Check sheet for the modelled part. Datum: model origin and axes. Units: mm. A direction names the side the tool comes from. Coordinates: 2 decimals unless noted, no trailing zeros. Write each loop counter-clockwise with the first axis right and the second up, starting at its lowest first coordinate (ties: lowest second). Pieces come first, ordered by that corner, then holes. Notation, with made-up numbers: (67.25, -38.75) -> (123.25, -38.75) arc R23 ccw to (123.25, -4.75) -> close; hole circle Ø11 at (-9, -38). An arc over 180 degrees is marked (long way). Put each result on its own line as item: value.
```python
from build123d import *

# Parameters (mm, degrees)
ESQUISSE1_W                  = 20
ESQUISSE1_H                  = 12
BOSS_EXTRU_1_DEPTH           = 15
ESQUISSE1_4_R                = 4.2
ENL_V_MAT_EXTRU_1_DEPTH      = 12
CONG_2_R                     = 4
ENL_V_MAT_EXTRU_2_DEPTH      = 54.749418763
ENL_V_MAT_EXTRU_2_DEPTH_BACK = 10
ESQUISSE2_R                  = 2.75
ESQUISSE4_R                  = 3.5
ENL_V_MAT_EXTRU_3_DEPTH      = 1
ESQUISSE5_R                  = 3.5
ENL_V_MAT_EXTRU_4_DEPTH      = 1
ENL_V_MAT_EXTRU_5_DEPTH      = 49.093658782
CONG_3_R                     = 10


with BuildPart() as part:
    # Esquisse1 → Boss.-Extru.1 (new body)
    with BuildSketch(Plane(origin=(0, 0, 0), x_dir=(1, 0, 0), z_dir=(0, 1, 0))):
        Polygon((-38, 12), (-42, 8), (-42, -8), (-38, -12), (38, -12), (42, -8), (42, 8), (38, 12), (22, 12), (14, 18), (-14, 18), (-22, 12), align=None)
        with Locations((0, 3)):
            Rectangle(ESQUISSE1_W, ESQUISSE1_H, mode=Mode.SUBTRACT)
    extrude(amount=BOSS_EXTRU_1_DEPTH)

    # Congé1
    # a fillet whose section is not a circle: 4 mm, written as the material it adds along each edge
    with BuildSketch(Plane(origin=(22, 0, -12), x_dir=(1, 0, 0), z_dir=(0, 1, 0)), Plane(origin=(-22, 0, -12), x_dir=(0.7999999999999996, 0, -0.6000000000000003), z_dir=(0, 1, 0))) as cong_1_piece_1:
        with BuildLine():
            add(Edge.make_bspline([(1.333333333, 0), (1.087283439, 0), (0.841233545, 0), (0.292751215, 0.037020099), (-0.211988912, 0.205266808), (-0.672986836, 0.504740127), (-0.869826751, 0.652370064), (-1.066666667, 0.8)], knots=[0, 0, 0, 0, 0, 0, 0.5, 0.5, 1, 1, 1, 1, 1, 1], degree=5))
            Line((-1.066666667, 0.8), (0, 0))
            Line((0, 0), (1.333333333, 0))
        make_face()
    extrude(amount=15)
    # a fillet whose section is not a circle: 4 mm, written as the material it takes off along each edge
    with BuildSketch(Plane(origin=(42, -4.142135624, 8), x_dir=(-0.707106781186547, 0, 0.7071067811865481), z_dir=(0, 1, 0)), Plane(origin=(38, -4.142135624, 12), x_dir=(-1, 0, 0), z_dir=(0, 1, 0)), Plane(origin=(42, -4.142135624, -8), x_dir=(0, 0, 1), z_dir=(0, 1, 0)), Plane(origin=(38, -4.142135624, -12), x_dir=(0.7071067811865481, 0, 0.707106781186547), z_dir=(0, 1, 0)), Plane(origin=(-42, -4.142135624, -8), x_dir=(0.7071067811865475, 0, -0.7071067811865475), z_dir=(0, 1, 0)), Plane(origin=(-42, -4.142135624, 8), x_dir=(0, 0, -1), z_dir=(0, 1, 0)), Plane(origin=(-38, -4.142135624, 12), x_dir=(-0.7071067811865465, 0, -0.7071067811865486), z_dir=(0, 1, 0))) as cong_1_2_piece_1:
        with BuildLine():
            add(Edge.make_bspline([(1.656854249, 0), (1.35356905, 0), (1.050283851, 0), (0.373674798, -0.056927592), (-0.223974097, -0.30448187), (-0.742662833, -0.742662833), (-0.957117854, -0.957117854), (-1.171572875, -1.171572875)], knots=[0, 0, 0, 0, 0, 0, 0.5, 0.5, 1, 1, 1, 1, 1, 1], degree=5))
            Line((-1.171572875, -1.171572875), (0, 0))
            Line((0, 0), (1.656854249, 0))
        make_face()
    extrude(amount=23.284271247, mode=Mode.SUBTRACT)
    with BuildSketch(Plane(origin=(14, -3.333333333, -18), x_dir=(0.7999999999999996, 0, 0.6000000000000003), z_dir=(0, 1, 0)), Plane(origin=(-14, -3.333333333, -18), x_dir=(1, 0, 0), z_dir=(0, 1, 0))) as cong_1_2_piece_2:
        with BuildLine():
            add(Edge.make_bspline([(1.333333333, 0), (1.087283439, 0), (0.841233545, 0), (0.292751215, -0.037020099), (-0.211988912, -0.205266808), (-0.672986836, -0.504740127), (-0.869826751, -0.652370064), (-1.066666667, -0.8)], knots=[0, 0, 0, 0, 0, 0, 0.5, 0.5, 1, 1, 1, 1, 1, 1], degree=5))
            Line((-1.066666667, -0.8), (0, 0))
            Line((0, 0), (1.333333333, 0))
        make_face()
    extrude(amount=21.666666667, mode=Mode.SUBTRACT)
    with BuildSketch(Plane(origin=(-38, -4.142135624, -12), x_dir=(-0.7071067811865465, 0, 0.7071067811865486), z_dir=(0, 1, 0))) as cong_1_2_piece_3:
        with BuildLine():
            add(Edge.make_bspline([(1.656854249, 0), (1.35356905, 0), (1.050283851, 0), (0.373674798, 0.056927592), (-0.223974097, 0.30448187), (-0.742662833, 0.742662833), (-0.957117854, 0.957117854), (-1.171572875, 1.171572875)], knots=[0, 0, 0, 0, 0, 0, 0.5, 0.5, 1, 1, 1, 1, 1, 1], degree=5))
            Line((-1.171572875, 1.171572875), (0, 0))
            Line((0, 0), (1.656854249, 0))
        make_face()
    extrude(amount=23.284271247, mode=Mode.SUBTRACT)

    # Esquisse1<4> → Enlèv. mat.-Extru.1 (cut)
    with BuildSketch(Plane(origin=(0, 0, 0), x_dir=(1, 0, 0), z_dir=(0, 1, 0))):
        with Locations(Location((-30, 0, 0), (0, 0, 270))):
            Circle(ESQUISSE1_4_R)
        with Locations(Location((30, 0, 0), (0, 0, 270))):
            Circle(ESQUISSE1_4_R)
    extrude(amount=ENL_V_MAT_EXTRU_1_DEPTH, mode=Mode.SUBTRACT)

    # Congé2
    cong_2_edges = [part.edges().sort_by_distance(p)[0] for p in [
        (-10, 7.5, -9),
        (-10, 7.5, 3),
        (10, 7.5, 3),
        (10, 7.5, -9),
    ]]
    fillet(cong_2_edges, radius=CONG_2_R)

    # Esquisse2 → Enlèv. mat.-Extru.2 (cut, two sides: drawn at the far end of the back side and taken through both)
    with BuildSketch(Plane.XY.offset(12).offset(-ENL_V_MAT_EXTRU_2_DEPTH_BACK)):
        with Locations(Location((-28.75, 7.5, 0), (0, 0, 180))):
            Circle(ESQUISSE2_R)
        with Locations(Location((28.75, 7.5, 0), (0, 0, 180))):
            Circle(ESQUISSE2_R)
    extrude(amount=ENL_V_MAT_EXTRU_2_DEPTH + ENL_V_MAT_EXTRU_2_DEPTH_BACK, mode=Mode.SUBTRACT)

    # Esquisse4 → Enlèv. mat.-Extru.3 (cut)
    with BuildSketch(Plane.XY.offset(12)):
        with Locations((28.75, 7.5)):
            Circle(ESQUISSE4_R)
    extrude(amount=-ENL_V_MAT_EXTRU_3_DEPTH, mode=Mode.SUBTRACT)

    # Esquisse5 → Enlèv. mat.-Extru.4 (cut)
    with BuildSketch(Plane.XY.offset(12)):
        with Locations((-28.75, 7.5)):
            Circle(ESQUISSE5_R)
    extrude(amount=-ENL_V_MAT_EXTRU_4_DEPTH, mode=Mode.SUBTRACT)

    # Esquisse6 → Enlèv. mat.-Extru.5 (cut, through all)
    with BuildSketch(Plane.XZ):
        Polygon((-23.333333333, -12), (-10, -5), (10, -5), (23.333333333, -12), (23.333333333, -18), (-23.333333333, -18), align=None)
    extrude(amount=-ENL_V_MAT_EXTRU_5_DEPTH, mode=Mode.SUBTRACT)

    # Congé3
    cong_3_edges = [part.edges().sort_by_distance(p)[0] for p in [
        (-23.333333333, 7.5, -12),
        (-10, 7.5, -5),
        (10, 7.5, -5),
        (23.333333333, 7.5, -12),
    ]]
    fillet(cong_3_edges, radius=CONG_3_R)


solid = part.part
```
Q1. Depth check by flat-ended pin: P1, Ø2.5, axis at x = -32, z = 0, coming from the -Y side; P2, Ø2, axis at x = -28.5, y = 9, coming from the +Z side. Enter the tip coordinate at first touch or a pass-through.
Recorded:
P1: stops at y = 12
P2: stops at z = -3.37
Q2. Cross-section at C-C (x = -0.5). Record the cut outline in (y, z), plus the area to 3 significant figures.
Recorded:
outline: (0, 3) -> (15, 3) -> (15, 12) -> (0, 12) -> close
area: 135 mm2
Q3. Material ranges on line 1 along Y through (x, z) = (-28.75, 11.4); line 2 along X through (y, z) = (8.25, 1.5); line 3 along X through (y, z) = (3, 0), recorded low to high.
Recorded:
line 1: y = 0 to 4, 11 to 15
line 2: x = -42 to -33.92, -26.08 to -9.12, 9.12 to 26.08, 33.92 to 42
line 3: x = -42 to -34.2, -25.8 to -9.87, 9.87 to 25.8, 34.2 to 42
Q4. Cross-section at B-B (z = 0.5). Record the cut outline in (x, y).
Recorded:
outline: (-42, 0) -> (-34.17, 0) -> (-34.17, 12) -> (-25.83, 12) -> (-25.83, 0) -> (-9.71, 0) -> (-9.71, 15) -> (-42, 15) -> close; (9.71, 0) -> (25.83, 0) -> (25.83, 12) -> (34.17, 12) -> (34.17, 0) -> (42, 0) -> (42, 15) -> (9.71, 15) -> close
Q5. Cross-section at A-A (x = -28.75). Record the cut outline in (y, z).
Recorded:
outline: (0, -12) -> (15, -12) -> (15, 12) -> (11, 12) -> (11, 11) -> (10.25, 11) -> (10.25, 4.01) -> (12, 4.01) -> (12, -4.01) -> (0, -4.01) -> close; (0, 4.01) -> (4.75, 4.01) -> (4.75, 11) -> (4, 11) -> (4, 12) -> (0, 12) -> close
Q6. Mould release check, pull along Y, two halves, no side actions. Record for faces 5 (the cylindrical face through (26.21, 8.55, 7.44)), 6 (the flat face through (26, 6, 11)), 7 (the flat face through (-40, 7, 10)), 8 (the flat face through (-30, 12, 0)): released by +Y, released by -Y, zero draft, split by the parting line, or undercut.
Recorded:
face 5: undercut
face 6: undercut
face 7: zero draft
face 8: released by -Y
Q7. Tool access check on faces 1 (the cylindrical face through (-8.634, 7.605, 2.01)), 2 (the flat face through (-1, 0, 5)), 3 (the flat face through (-27, 5, 11)), 4 (the cylindrical face through (-32.6, 5.9, -3.3)). Record the directions out of +Z, -Z, +X, -X, +Y, -Y that give a thin tool (end or side, any length) a straight path to the whole face; none if there is none.
Recorded:
face 1: -Z, +Y, -Y
face 2: +Z, -Z, +X, -X, -Y
face 3: +Z
face 4: -Y
